CAD build for the part. Positions are in the model's coordinates, mm. A direction names the side the tool comes from. Coordinates: 2 decimals unless noted, no trailing zeros. Write each loop counter-clockwise with the first axis right and the second up, starting at its lowest first coordinate (ties: lowest second). Pieces come first, ordered by that corner, then holes. Notation, with made-up numbers: (34.5, 6.25) - (41.5, 6.25) arc R16 ccw to (41.5, 37.25) - close; hole circle Ø3 at (-30, 64.5). An arc over 180 degrees is marked (long way). Answer in a Markdown table with one row per item. Add a question column.
Q1. Pin check, flat tips, straight feed: pin 1 (9 mm diameter, centred on x = -12, z = 9, fed in from +Y); pin 2 (8 mm diameter, centred on x = -14, z = -10.5, fed in from +Y); pin 3 (16.5 mm diameter, centred on y = 16.5, z = -6, fed in from -X); pin 4 (6 mm diameter, centred on x = -12, z = -9, fed in from -Y). Stop position of each tip, or through.
Q2. 3-axis set-ups, long thin cutter, end or side, ignore diameter. For faces 5 (the flat face through (3.007, 15.32, 11.772)), 6 (the cylindrical face through (11.58, 1.97, 3)), 7 (the flat face through (-4.5, 37, 16)): which of +Z, -Z, +X, -X, +Y, -Y reach the whole face in a straight line?
Q3. Two-plate mould, pull along Z, no slides. Class faces 1 (the cylindrical face through (15.85, 3.94, 13.93)), 2 (the flat face through (-9.8, 7.4, 11.2)), 3 (the cylindrical face through (-9.38, 3.65, -9.83)), 4 (the flat face through (17.5, 4, 0)): +Z half, -Z half, draft (parallel to the pull), parting line (faces both ways), or undercut.
Q4. Band-saw the part on A-A (x = -1.5). List the corners of the cut face in (y, z).
Q5. Band-saw the part on C-C (z = -9). List the corners of the cut face in (x, y), and give its area (3 significant figures).
Q6. Band-saw the part on D-D (y = 33.5). List the corners of the cut face in (x, z).
Q7. Drill centre lines: line 1 along X through (y, z) = (7.6, 9); line 2 along X through (y, z) = (4.5, 9); line 3 along X through (y, z) = (9.5, 11). Where is each one in solid material? Low to high. Write a range as from..to.
Q8. Band-saw the part on B-B (y = 5.5). List the corners of the cut face in (x, z), and give its area (3 significant figures).
```python
from build123d import *

# Parameters (mm, degrees)
SKETCH1_R                = 2.75
BOSS_EXTRUDE1_DEPTH      = 8
BOSS_EXTRUDE2_DEPTH      = 3.5
BOSS_EXTRUDE2_DEPTH_BACK = 3.5
CUT_EXTRUDE1_DEPTH       = 1
CUT_EXTRUDE2_DEPTH       = 1
CUT_EXTRUDE3_DEPTH       = 4
SKETCH7_R                = 5
CUT_EXTRUDE4_DEPTH       = 0.6
SKETCH8_R                = 5
CUT_EXTRUDE5_DEPTH       = 0.6
SKETCH9_R                = 5
CUT_EXTRUDE6_DEPTH       = 0.6
SKETCH10_R               = 5
CUT_EXTRUDE7_DEPTH       = 0.6


with BuildPart() as part:
    # Sketch1 → Boss-Extrude1 (new body)
    with BuildSketch(Plane(origin=(0, 0, 0), x_dir=(1, 0, 0), z_dir=(0, 1, 0))):
        with BuildLine():
            Line((-12, -15.5), (12, -15.5))
            ThreePointArc((12, -15.5), (15.889087297, -13.889087297), (17.5, -10))
            Line((17.5, -10), (17.5, 10))
            ThreePointArc((17.5, 10), (15.889087297, 13.889087297), (12, 15.5))
            Line((12, 15.5), (-12, 15.5))
            ThreePointArc((-12, 15.5), (-15.889087297, 13.889087297), (-17.5, 10))
            Line((-17.5, 10), (-17.5, -10))
            ThreePointArc((-17.5, -10), (-15.889087297, -13.889087297), (-12, -15.5))
        make_face()
        with Locations((12, 9)):
            Circle(SKETCH1_R, mode=Mode.SUBTRACT)
        with Locations((12, -9)):
            Circle(SKETCH1_R, mode=Mode.SUBTRACT)
        with Locations((-12, 9)):
            Circle(SKETCH1_R, mode=Mode.SUBTRACT)
        with Locations((-12, -9)):
            Circle(SKETCH1_R, mode=Mode.SUBTRACT)
    extrude(amount=BOSS_EXTRUDE1_DEPTH)

    # Sketch2 → Boss-Extrude2 (add, two sides)
    with BuildSketch(Plane(origin=(0, 0, 0), x_dir=(0, 0, -1), z_dir=(1, 0, 0))) as boss_extrude2_sk:
        with BuildLine():
            Line((-21.65714117, 30.903921337), (-15.5, 8))
            Line((-15.5, 8), (15.5, 8))
            Line((15.5, 8), (-3.491565957, 38.754193576))
            ThreePointArc((-3.491565957, 38.754193576), (-8.033064713, 24.320488879), (-21.65714117, 30.903921337))
        make_face()
    extrude(amount=BOSS_EXTRUDE2_DEPTH)
    extrude(boss_extrude2_sk.sketch, amount=-BOSS_EXTRUDE2_DEPTH_BACK)

    # Sketch3 → Cut-Extrude1 (cut)
    with BuildSketch(Plane(origin=(3.5, 0, 0), x_dir=(0, 0, -1), z_dir=(1, 0, 0))):
        with BuildLine():
            Line((-13.298775285, 20.997472945), (-10.202804209, 9.480784267))
            ThreePointArc((-10.202804209, 9.480784267), (-9.48825077, 8.412796254), (-8.271375975, 8))
            Line((-8.271375975, 8), (5.450161602, 8))
            ThreePointArc((5.450161602, 8), (7.196826629, 9.025750912), (7.151848411, 11.050838715))
            Line((7.151848411, 11.050838715), (-2.004518147, 25.878297925))
            ThreePointArc((-2.004518147, 25.878297925), (-3.452381431, 26.811287231), (-5.088504172, 26.272882634))
            ThreePointArc((-5.088504172, 26.272882634), (-8.03306474, 24.320488867), (-11.47278921, 23.513907231))
            ThreePointArc((-11.47278921, 23.513907231), (-12.986087496, 22.691286214), (-13.298775285, 20.997472945))
        make_face()
    extrude(amount=-CUT_EXTRUDE1_DEPTH, mode=Mode.SUBTRACT)

    # Sketch4 → Cut-Extrude2 (cut)
    with BuildSketch(Plane(origin=(-3.5, 0, 0), x_dir=(0, 0, -1), z_dir=(1, 0, 0))):
        with BuildLine():
            Line((-13.298775285, 20.997472945), (-10.202804209, 9.480784267))
            ThreePointArc((-10.202804209, 9.480784267), (-9.48825077, 8.412796254), (-8.271375975, 8))
            Line((-8.271375975, 8), (5.450161602, 8))
            ThreePointArc((5.450161602, 8), (7.196826629, 9.025750912), (7.151848411, 11.050838715))
            Line((7.151848411, 11.050838715), (-2.004518147, 25.878297925))
            ThreePointArc((-2.004518147, 25.878297925), (-3.452381431, 26.811287231), (-5.088504172, 26.272882634))
            ThreePointArc((-5.088504172, 26.272882634), (-8.03306474, 24.320488867), (-11.47278921, 23.513907231))
            ThreePointArc((-11.47278921, 23.513907231), (-12.986087496, 22.691286214), (-13.298775285, 20.997472945))
        make_face()
    extrude(amount=CUT_EXTRUDE2_DEPTH, mode=Mode.SUBTRACT)

    # Sketch5 → Revolve1 (revolve)
    with BuildSketch(Plane.XY.offset(12)):
        with BuildLine():
            Line((-4.5, 42.5), (-4.5, 38.5))
            Line((-4.5, 38.5), (4.5, 38.5))
            Line((4.5, 38.5), (4.5, 42.5))
            ThreePointArc((4.5, 42.5), (4.207106781, 43.207106781), (3.5, 43.5))
            Line((3.5, 43.5), (-3.5, 43.5))
            ThreePointArc((-3.5, 43.5), (-4.207106781, 43.207106781), (-4.5, 42.5))
        make_face()
    revolve(axis=Axis((4.5, 33.5, 12), (-1, 0, 0)))

    # Sketch6 → Cut-Extrude3 (cut)
    with BuildSketch(Plane(origin=(0, 0, 0), x_dir=(1, 0, 0), z_dir=(0, 1, 0))):
        with BuildLine():
            Line((-12, 1.771583853), (-12, -1.771583853))
            ThreePointArc((-12, -1.771583853), (-11.591644792, -2.982644073), (-10.533333143, -3.699161545))
            ThreePointArc((-10.533333143, -3.699161545), (-7.855282825, -5.384572011), (-6.549108126, -8.266666667))
            ThreePointArc((-6.549108126, -8.266666667), (-5.883526804, -9.505545305), (-4.566965626, -10))
            Line((-4.566965626, -10), (4.566965626, -10))
            ThreePointArc((4.566965626, -10), (5.883526804, -9.505545305), (6.549108126, -8.266666667))
            ThreePointArc((6.549108126, -8.266666667), (7.85528289, -5.384571937), (10.533333333, -3.699161492))
            ThreePointArc((10.533333333, -3.699161492), (11.591644852, -2.982643994), (12, -1.771583853))
            Line((12, -1.771583853), (12, 1.771583853))
            ThreePointArc((12, 1.771583853), (11.591644852, 2.982643994), (10.533333333, 3.699161492))
            ThreePointArc((10.533333333, 3.699161492), (7.85528289, 5.384571937), (6.549108126, 8.266666667))
            ThreePointArc((6.549108126, 8.266666667), (5.883526804, 9.505545305), (4.566965626, 10))
            Line((4.566965626, 10), (-4.566965626, 10))
            ThreePointArc((-4.566965626, 10), (-5.883526804, 9.505545305), (-6.549108126, 8.266666667))
            ThreePointArc((-6.549108126, 8.266666667), (-7.855282955, 5.384571863), (-10.533333524, 3.699161439))
            ThreePointArc((-10.533333524, 3.699161439), (-11.591644911, 2.982643916), (-12, 1.771583853))
        make_face()
    extrude(amount=CUT_EXTRUDE3_DEPTH, mode=Mode.SUBTRACT)

    # Sketch7 → Cut-Extrude4 (cut)
    with BuildSketch(Plane(origin=(0, 8, 0), x_dir=(1, 0, 0), z_dir=(0, 1, 0))):
        with Locations((12, 9)):
            Circle(SKETCH7_R)
    extrude(amount=-CUT_EXTRUDE4_DEPTH, mode=Mode.SUBTRACT)

    # Sketch8 → Cut-Extrude5 (cut)
    with BuildSketch(Plane(origin=(0, 8, 0), x_dir=(1, 0, 0), z_dir=(0, 1, 0))):
        with Locations((-12, 9)):
            Circle(SKETCH8_R)
    extrude(amount=-CUT_EXTRUDE5_DEPTH, mode=Mode.SUBTRACT)

    # Sketch9 → Cut-Extrude6 (cut)
    with BuildSketch(Plane(origin=(0, 8, 0), x_dir=(1, 0, 0), z_dir=(0, 1, 0))):
        with Locations((12, -9)):
            Circle(SKETCH9_R)
    extrude(amount=-CUT_EXTRUDE6_DEPTH, mode=Mode.SUBTRACT)

    # Sketch10 → Cut-Extrude7 (cut)
    with BuildSketch(Plane(origin=(0, 8, 0), x_dir=(1, 0, 0), z_dir=(0, 1, 0))):
        with Locations((-12, -9)):
            Circle(SKETCH10_R)
    extrude(amount=-CUT_EXTRUDE7_DEPTH, mode=Mode.SUBTRACT)


solid = part.part
```
Checked values:
| question | item | result |
|---|---|---|
| 1 | pin 1 | stops at y = 7.4 |
| 1 | pin 2 | stops at y = 8 |
| 1 | pin 3 | stops at x = -3.5 |
| 1 | pin 4 | stops at y = 0 |
| 2 | face 5 | +X |
| 2 | face 6 | -Y |
| 2 | face 7 | +Z, -Z, -X, +Y |
| 3 | face 1 | +Z half |
| 3 | face 2 | undercut |
| 3 | face 3 | undercut |
| 3 | face 4 | draft |
| 4 | outline | (0, -15.5) - (8, -15.5) - (38.75, 3.49) arc R10 ccw to (30.9, 21.66) - (8, 15.5) - (0, 15.5) - (0, 10) - (4, 10) - (4, -10) - (0, -10) - close; hole circle Ø10 at (33.5, 12) |
| 5 | outline | (-17.5, 0) - (-14.75, 0) - (-14.75, 7.4) - (-17, 7.4) - (-17, 8) - (-17.5, 8) - close; (-9.25, 0) - (-6.3, 0) - (-6.3, 4) - (6.3, 4) - (6.3, 0) - (9.25, 0) - (9.25, 7.4) - (7, 7.4) - (7, 8) - (3.5, 8) - (3.5, 18.53) - (-3.5, 18.53) - (-3.5, 8) - (-7, 8) - (-7, 7.4) - (-9.25, 7.4) - close; (14.75, 0) - (17.5, 0) - (17.5, 8) - (17, 8) - (17, 7.4) - (14.75, 7.4) - close |
| 5 | area | 210 mm² |
| 6 | outline | (-4.5, 3) arc R1 ccw to (-3.5, 2) - (-3.5, 0.25) - (3.5, 0.25) - (3.5, 2) arc R1 ccw to (4.5, 3) - (4.5, 7) - (-4.5, 7) - close; (-4.5, 17) - (4.5, 17) - (4.5, 21) arc R1 ccw to (3.5, 22) - (-3.5, 22) arc R1 ccw to (-4.5, 21) - close |
| 7 | line 1 | x = -17.5..-17, -7..7, 17..17.5 |
| 7 | line 2 | x = -17.5..-14.75, -9.25..9.25, 14.75..17.5 |
| 7 | line 3 | x = -3.5..3.5 |
| 8 | outline | (-17.5, -10) arc R5.5 ccw to (-12, -15.5) - (12, -15.5) arc R5.5 ccw to (17.5, -10) - (17.5, 10) arc R5.5 ccw to (12, 15.5) - (-12, 15.5) arc R5.5 ccw to (-17.5, 10) - close; hole circle Ø5.5 at (-12, -9); hole circle Ø5.5 at (-12, 9); hole circle Ø5.5 at (12, -9); hole circle Ø5.5 at (12, 9) |
| 8 | area | 964 mm² |
